Build history of the part. All positions in model axes, mm. Face numbers are marked on the shaded views. A direction names the side the tool comes from. Give positions to 0.01 mm unless a question says otherwise; leave off trailing zeros. Order: outer loops, then holes, each group sorted by start corner. A loop starts at its lowest first (then second) coordinate and runs counter-clockwise, first axis right, second up. Notation, with made-up numbers: (3.5, 59.25) - (21.5, 59.25) arc R29 cw to (21.5, 95.25) - close; hole circle Ø4 at (62, -2). An arc over 180 degrees is marked (long way). Use a Markdown table: item, result.
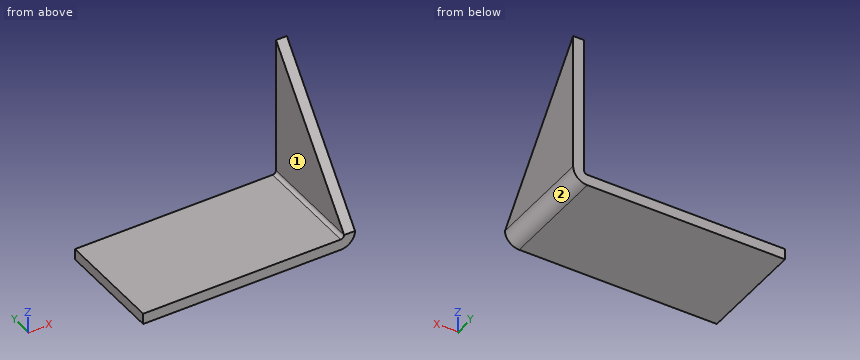
from build123d import *

# Parameters (mm, degrees)
SKETCH2_W               = 57.912
SKETCH2_H               = 31.75
BASE_FLANGE1_DEPTH      = 3.175
EDGE_FLANGE1_DEPTH      = 31.75
CUT_EXTRUDE2_DEPTH      = 78.991112917
CUT_EXTRUDE2_DEPTH_BACK = 3.175


# Sheet-metal steps are written as plain solids
with BuildPart() as part:
    # Sketch2 → Base-Flange1 (new body)
    with BuildSketch(Plane.XY):
        Rectangle(SKETCH2_W, SKETCH2_H)
    extrude(amount=BASE_FLANGE1_DEPTH)

    # Edge-Flange1 section (across the edge) → Edge-Flange1 (add)
    with BuildSketch(Plane(origin=(29.956, -15.875, 3.175), x_dir=(-1, 0, 0), z_dir=(0, 1, 0))):
        with BuildLine():
            Line((-3.175, 1), (-3.175, 41.275))
            Line((-3.175, 41.275), (0, 41.275))
            Line((0, 41.275), (0, 1))
            ThreePointArc((0, 1), (0.292893219, 0.292893219), (1, 0))
            Line((1, 0), (1, -3.175))
            ThreePointArc((1, -3.175), (-1.952170811, -1.952170811), (-3.175, 1))
        make_face()
    extrude(amount=EDGE_FLANGE1_DEPTH)

    # Sketch11 → Cut-Extrude2 (cut, two sides: drawn at the far end of the back side and taken through both)
    with BuildSketch(Plane(origin=(33.131, 0, 0), x_dir=(0, 0, -1), z_dir=(1, 0, 0)).offset(-CUT_EXTRUDE2_DEPTH_BACK)):
        Polygon((89.473958122, -89.701304665), (-4.175, -15.875), (-44.45, 15.875), (-138.098958122, 89.701304665), (-285.751567452, -97.596611579), (-58.178651208, -276.999220909), align=None)
    extrude(amount=CUT_EXTRUDE2_DEPTH + CUT_EXTRUDE2_DEPTH_BACK, mode=Mode.SUBTRACT)


solid = part.part
1) Slice it at B-B (x = 26.5). Write the cut outline in (y, z) (3 decimals), and give its area (3 significant figures).
Computed:
| item | result |
|---|---|
| outline | (-15.875, 0) - (15.875, 0) - (15.875, 3.175) - (-15.875, 3.175) - close |
| area | 101 mm² |
2) Pin check, flat tips, straight feed: P1, Ø12, axis at y = 1, z = 26, coming from the -X side; P2, Ø10, axis at x = 16.5, y = 9.5, coming from the +Z side (3 decimals); P3, Ø3, axis at x = 18, y = -3, coming from the -Z side; P4, Ø8, axis at y = -8.5, z = 24, coming from the +X side. Stop position of each tip, or through.
Computed:
| item | result |
|---|---|
| P1 | stops at x = 29.96 |
| P2 | stops at z = 3.175 |
| P3 | stops at z = 0 |
| P4 | passes through |
3) Wall check: line 1 (X direction, y = -1, z = 16); line 2 (Z direction, x = -13, y = -13) (3 decimals); line 3 (Y direction, x = 30, z = 42.5) (3 decimals). Give the ranges that are in metal, low to high. Write a range as from..to.
Computed:
| item | result |
|---|---|
| line 1 | x = 29.96..33.13 |
| line 2 | z = 0..3.175 |
| line 3 | y = 14.338..15.875 |
4) Slice it at C-C (z = 35). Write the cut outline in (x, y) (3 decimals).
Computed:
| item | result |
|---|---|
| outline | (29.956, 8.425) - (33.131, 8.425) - (33.131, 15.875) - (29.956, 15.875) - close |
5) Tool access for the marked faces 1 and 2: list every direction of +Z, -Z, +X, -X, +Y, -Y with a clear straight run to the whole face (end or side of a thin tool).
Computed:
| item | result |
|---|---|
| face 1 | +Z, -X, +Y, -Y |
| face 2 | -Z, +X, +Y, -Y |
6) Slice it at A-A (y = -12.5). Write the cut outline in (x, z) (3 decimals).
Computed:
| item | result |
|---|---|
| outline | (-28.956, 0) - (28.956, 0) arc R4.175 ccw to (33.131, 4.175) - (33.131, 8.456) - (29.956, 8.456) - (29.956, 4.175) arc R1 cw to (28.956, 3.175) - (-28.956, 3.175) - close |
7) Slice it at D-D (y = -7). Write the cut outline in (x, z) (3 decimals).
Computed:
| item | result |
|---|---|
| outline | (-28.956, 0) - (28.956, 0) arc R4.175 ccw to (33.131, 4.175) - (33.131, 15.433) - (29.956, 15.433) - (29.956, 4.175) arc R1 cw to (28.956, 3.175) - (-28.956, 3.175) - close |
